Work out the finished part from the listing and answer in its coordinate system (mm). Face numbers are marked on the shaded views. A direction names the side the tool comes from. Round coordinates to 2 decimals unless told otherwise and drop trailing zeros. Order: outer loops, then holes, each group sorted by start corner. A loop starts at its lowest first (then second) coordinate and runs counter-clockwise, first axis right, second up.
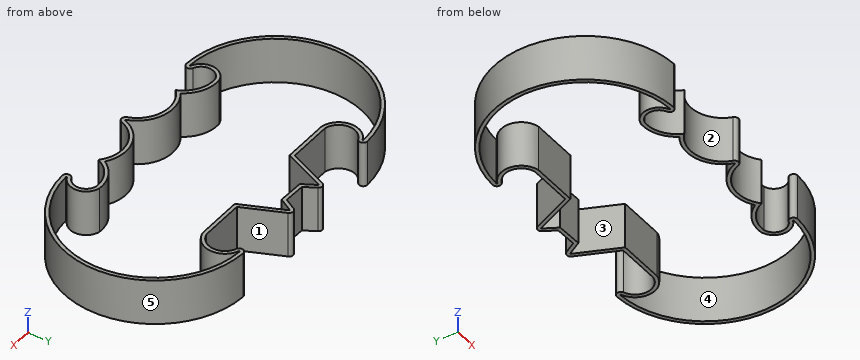
from build123d import *

# Parameters (mm, degrees)
F1_DEPTH = 10


with BuildPart() as f1:
    # F0 (on Top) → F1 (new body)
    with BuildSketch(Plane.XY):
        with BuildLine():
            ThreePointArc((-6.714271, -16.914273), (-0.235273, -15.199649), (4.738337, -19.691927))
            ThreePointArc((4.738337, -19.691927), (5.586952, -20.29217), (6.435566, -19.691927))
            ThreePointArc((6.435566, -19.691927), (11.409176, -15.199649), (17.888174, -16.914273))
            ThreePointArc((17.888174, -16.914273), (20.536513, -13.803613), (24.507416, -12.843491))
            ThreePointArc((24.507416, -12.843491), (26.536414, -15.25895), (24.919216, -17.967445))
            ThreePointArc((24.919216, -17.967445), (24.4038, -18.991339), (25.311912, -19.690872))
            ThreePointArc((25.311912, -19.690872), (44.486815, 0.074047), (25.459012, 19.98062))
            ThreePointArc((25.459012, 19.98062), (24.539987, 19.261705), (25.10301, 18.23972))
            ThreePointArc((25.10301, 18.23972), (27.400825, 14.613237), (24.559428, 11.394885))
            Line((24.559428, 11.394885), (14.999758, 11.394885))
            Line((14.999758, 11.394885), (11.213153, 20.033227))
            ThreePointArc((11.213153, 20.033227), (10.436556, 20.570639), (9.607449, 20.118428))
            Line((9.607449, 20.118428), (8.193074, 17.643271))
            Line((8.193074, 17.643271), (3.569399, 17.76631))
            Line((3.569399, 17.76631), (2.140906, 20.266173))
            ThreePointArc((2.140906, 20.266173), (1.311799, 20.718384), (0.535203, 20.180972))
            Line((0.535203, 20.180972), (-3.251402, 11.54263))
            Line((-3.251402, 11.54263), (-12.811073, 11.54263))
            ThreePointArc((-12.811073, 11.54263), (-15.638403, 14.619541), (-13.616246, 18.276324))
            ThreePointArc((-13.616246, 18.276324), (-13.125555, 19.299533), (-14.026369, 19.989655))
            ThreePointArc((-14.026369, 19.989655), (-33.31297, 0.203497), (-14.138009, -19.690872))
            ThreePointArc((-14.138009, -19.690872), (-13.229897, -18.991339), (-13.745313, -17.967445))
            ThreePointArc((-13.745313, -17.967445), (-15.362511, -15.25895), (-13.333513, -12.843491))
            ThreePointArc((-13.333513, -12.843491), (-9.36261, -13.803613), (-6.714271, -16.914273))
        make_face()
        with BuildLine():
            ThreePointArc((-14.110806, -18.891334), (-32.512973, 0.201246), (-14.003666, 19.189977))
            ThreePointArc((-14.003666, 19.189977), (-13.903576, 19.113297), (-13.958097, 18.999607))
            ThreePointArc((-13.958097, 18.999607), (-16.427445, 14.482007), (-12.888596, 10.74263))
            Line((-12.888596, 10.74263), (-2.728596, 10.74263))
            Line((-2.728596, 10.74263), (1.2679, 19.859795))
            ThreePointArc((1.2679, 19.859795), (1.354189, 19.919508), (1.446312, 19.869262))
            Line((1.446312, 19.869262), (3.098136, 16.978568))
            Line((3.098136, 16.978568), (8.650219, 16.830822))
            Line((8.650219, 16.830822), (10.302044, 19.721517))
            ThreePointArc((10.302044, 19.721517), (10.394167, 19.771763), (10.480455, 19.71205))
            Line((10.480455, 19.71205), (14.476952, 10.594885))
            Line((14.476952, 10.594885), (24.636952, 10.594885))
            ThreePointArc((24.636952, 10.594885), (28.19471, 14.507176), (25.386326, 18.987873))
            ThreePointArc((25.386326, 18.987873), (25.323767, 19.101427), (25.425881, 19.181307))
            ThreePointArc((25.425881, 19.181307), (43.686821, 0.077013), (25.284709, -18.891334))
            ThreePointArc((25.284709, -18.891334), (25.183808, -18.813608), (25.241076, -18.699842))
            ThreePointArc((25.241076, -18.699842), (27.330713, -15.158302), (24.636952, -12.051417))
            ThreePointArc((24.636952, -12.051417), (20.608667, -12.845247), (17.621218, -15.661696))
            ThreePointArc((17.621218, -15.661696), (10.711949, -14.563871), (5.681242, -19.425476))
            ThreePointArc((5.681242, -19.425476), (5.586952, -19.49217), (5.492661, -19.425476))
            ThreePointArc((5.492661, -19.425476), (0.461954, -14.563871), (-6.447315, -15.661696))
            ThreePointArc((-6.447315, -15.661696), (-9.434764, -12.845247), (-13.463048, -12.051417))
            ThreePointArc((-13.463048, -12.051417), (-16.15681, -15.158302), (-14.067173, -18.699842))
            ThreePointArc((-14.067173, -18.699842), (-14.009905, -18.813608), (-14.110806, -18.891334))
        make_face(mode=Mode.SUBTRACT)
    extrude(amount=F1_DEPTH)


solid = f1.part
Item 1: A tool of negligible diameter and unlimited length cuts with its end or side. For the marked faces 1, 2 and 3, from which of +Z, -Z, +X, -X, +Y, -Y can it reach the whole face along a straight path? Write none if from no direction.
Item 2: Given pin 1 (5 mm diameter, centred on x = 18.5, z = 6.5, fed in from +Y); pin 2 (5 mm diameter, centred on x = -6, z = 4, fed in from +Y); pin 3 (1.5 mm diameter, centred on y = 2, z = 4, fed in from +X), each flat-ended and moving along its own axis, determine where each tip first touches the part or whether it passes through.
Item 3: Find section A-A (y = 1.5). Write down the section's boundary in (x, z).
Item 4: Find the intervals of material crossed by line 1 along Y through (x, z) = (23.5, 1); line 2 along Y through (x, z) = (9, 5.25); line 3 along X through (y, z) = (8.5, 7.5), in increasing order.
Item 5: For a pull along X with two mould halves and no side action, classify the marked faces 4 and 5 as released by +X, released by -X, zero draft, split by the parting line, or undercut.
Item 6: Find section B-B (x = -28). Write down the section's boundary in (y, z).
Model answer:
1. face 1: +Z, -Z, +Y
1. face 2: +Z, -Z, -Y
1. face 3: +Z, -Z
2. pin 1: stops at y = 11.39
2. pin 2: stops at y = 11.54
2. pin 3: stops at x = 44.46
3. outline: (-33.27, 0) - (-32.46, 0) - (-32.46, 10) - (-33.27, 10) - close; (43.64, 0) - (44.44, 0) - (44.44, 10) - (43.64, 10) - close
4. line 1: y = -12.84 to -12.04, 10.59 to 11.39
4. line 2: y = -16.3 to -15.34, 17.44 to 19.06
4. line 3: x = -31.47 to -30.58, 41.76 to 42.64
5. face 4: undercut
5. face 5: released by +X
6. outline: (-13.37, 0) - (-12.16, 0) - (-12.16, 10) - (-13.37, 10) - close; (12.46, 0) - (13.66, 0) - (13.66, 10) - (12.46, 10) - close
